Can you work these out from the model? Positions are in its coordinate system, mm. A direction names the side the tool comes from. Give positions to 0.01 mm unless a question says otherwise; leave off trailing zeros. Loops run counter-clockwise (first coordinate to the right, second up) from the corner with the lowest first, then second, coordinate; pieces in that order, holes last. Notation, with made-up numbers: M -16,61 L 34,61 A25 cw 34,98 Z; hole C 76.5,-24 d2. An arc over 180 degrees is marked long. Answer as a JSON object with one key per item and string values.
```python
from build123d import *

# Parameters (mm, degrees)
SKETCH_1_W          = 15
SKETCH_1_H          = 15
EXTRUDE_1_DEPTH     = 410
SKETCH_2_W          = 11
SKETCH_2_H          = 11
CUT_EXTRUDE_1_DEPTH = 410
SKETCH_3_R          = 2.5
CUT_EXTRUDE_2_DEPTH = 15
SKETCH_4_R          = 1.5
CUT_EXTRUDE_3_DEPTH = 15


with BuildPart() as part:
    # 草图1 → 凸台-拉伸1 (new body)
    with BuildSketch(Plane(origin=(0, 0, 0), x_dir=(1, 0, 0), z_dir=(0, 1, 0))):
        Rectangle(SKETCH_1_W, SKETCH_1_H)
    extrude(amount=EXTRUDE_1_DEPTH)

    # 草图2 → 切除-拉伸1 (cut)
    with BuildSketch(Plane(origin=(0, 410, 0), x_dir=(1, 0, 0), z_dir=(0, 1, 0))):
        Rectangle(SKETCH_2_W, SKETCH_2_H)
    extrude(amount=-CUT_EXTRUDE_1_DEPTH, mode=Mode.SUBTRACT)

    # 草图3 → 切除-拉伸2 (cut)
    with BuildSketch(Plane.XY.offset(7.5)):
        with Locations((0, 85)):
            Circle(SKETCH_3_R)
        with Locations((0, 165)):
            Circle(SKETCH_3_R)
        with Locations((0, 245)):
            Circle(SKETCH_3_R)
        with Locations((0, 325)):
            Circle(SKETCH_3_R)
    extrude(amount=-CUT_EXTRUDE_2_DEPTH, mode=Mode.SUBTRACT)

    # 草图4 → 切除-拉伸3 (cut)
    with BuildSketch(Plane.ZY.offset(7.5)):
        with Locations((0, 12.5)):
            Circle(SKETCH_4_R)
        with Locations((0, 397.5)):
            Circle(SKETCH_4_R)
    extrude(amount=-CUT_EXTRUDE_3_DEPTH, mode=Mode.SUBTRACT)


solid = part.part
```
1) For faces 1 (the flat face through (0, 208, -5.5)), 2 (the flat face through (-7.5, 202, 0)), which set-ups out of +Z, -Z, +X, -X, +Y, -Y let a thin tool reach every point of the face, with its end or its side?
Answer list:
{"face 1": "+Y, -Y", "face 2": "+Z, -Z, -X, +Y, -Y"}
2) If we mould it in two halves opening along Z, with no side actions, what happens to faces 3 (the flat face through (0, 202, 7.5)), 4 (the flat face through (-7, 410, 0)), 5 (the flat face through (0, 208, 5.5))? For each: +Z half, -Z half, draft (parallel to the pull), parting line (faces both ways), or undercut.
Answer list:
{"face 3": "+Z half", "face 4": "draft", "face 5": "undercut"}
3) Suppose I cut it at A-A, the plane y = 191. Write out the boundary of the cut face in (x, z).
Answer list:
{"outline": "M -7.5,-7.5 L 7.5,-7.5 L 7.5,7.5 L -7.5,7.5 Z; hole M -5.5,-5.5 L 5.5,-5.5 L 5.5,5.5 L -5.5,5.5 Z"}
4) Suppose I cut it at B-B, the plane x = 0. Give the number of separate pieces and of enclosed holes in the cut face, and give its area (3 significant figures).
Answer list:
{"separate pieces": "10", "enclosed holes": "0", "area": "1,560 mm^2"}
5) Please list where these lines run through material, in increasing order: line 1 along Y through (x, z) = (0, -6.7); line 2 along Y through (x, z) = (-6.2, 0); line 3 along Z through (x, y) = (-2.5, 148). Write a range as from..to.
Answer list:
{"line 1": "0..82.5, 87.5..162.5, 167.5..242.5, 247.5..322.5, 327.5..410", "line 2": "0..11, 14..396, 399..410", "line 3": "-7.5..-5.5, 5.5..7.5"}
